Answer from the drawing. Dimensions are ordinates in mm from the lowest x, y and z of the part. Coordinates: 2 decimals unless noted, no trailing zeros. Order: outer loops, then holes, each group sorted by start corner. A loop starts at its lowest first (then second) coordinate and runs counter-clockwise, first axis right, second up. Notation, with made-up numbers: (35.5, 42) - (79.5, 42) arc R13 ccw to (79.5, 67) - close; hole circle Ø6 at (64, -34.5). An arc over 180 degrees is marked (long way). Use a Markdown table: item, result. Add a question column.
Item 1: Find the intervals of material crossed by line 1 along Z through (x, y) = (43, 1.25); line 2 along Z through (x, y) = (40.35, 1.55); line 3 along X through (y, z) = (1.85, 28.5), in increasing order.
Item 2: The part is cut by section B-B, the plane x = 7.45. Give the vertices of the cut face in (y, z).
Item 3: A flat-ended cylindrical pin translates along its axis: P1, Ø3.5, axis at x = 40.35, z = 12.41, coming from the -Y side. Find the tip coordinate at first contact, or state that the pin passes through.
Item 4: The part is cut by section A-A, the plane z = 25. Give the vertices of the cut face in (x, y), then the cut area to 3 significant figures.
Item 5: The part is cut by section D-D, the plane y = 0.95. State how many separate pieces and enclosed holes the cut face has, then the cut area to 3 significant figures.
Item 6: The part is cut by section C-C, the plane x = 31. Give the vertices of the cut face in (y, z).
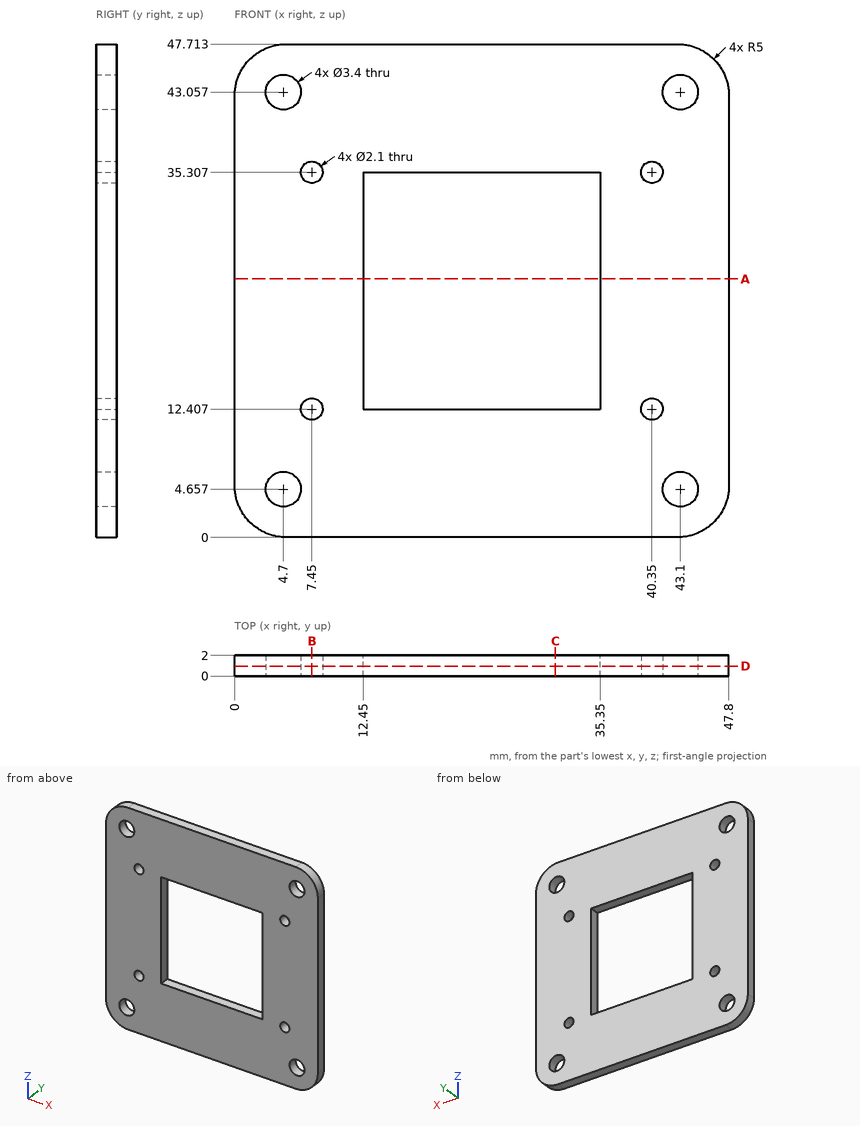
Solution:
| question | item | result |
|---|---|---|
| 1 | line 1 | z = 0 to 2.96, 6.35 to 41.36, 44.75 to 47.71 |
| 1 | line 2 | z = 0 to 11.36, 13.46 to 34.26, 36.36 to 47.71 |
| 1 | line 3 | x = 0 to 12.45, 35.35 to 47.8 |
| 2 | outline | (0, 0) - (2, 0) - (2, 11.36) - (0, 11.36) - close; (0, 13.46) - (2, 13.46) - (2, 34.26) - (0, 34.26) - close; (0, 36.36) - (2, 36.36) - (2, 47.71) - (0, 47.71) - close |
| 3 | P1 | stops at y = 0 |
| 4 | outline | (0, 0) - (12.45, 0) - (12.45, 2) - (0, 2) - close; (35.35, 0) - (47.8, 0) - (47.8, 2) - (35.35, 2) - close |
| 4 | area | 49.8 mm2 |
| 5 | separate pieces | 1 |
| 5 | enclosed holes | 9 |
| 5 | area | 1,680 mm2 |
| 6 | outline | (0, 0) - (2, 0) - (2, 12.41) - (0, 12.41) - close; (0, 35.31) - (2, 35.31) - (2, 47.71) - (0, 47.71) - close |
